```python
from build123d import *

# Parameters (mm, degrees)
SKETCH1_R           = 2.25
BOSS_EXTRUDE1_DEPTH = 30
SKETCH2_R           = 3.5
BOSS_EXTRUDE2_DEPTH = 2
BOSS_EXTRUDE2_TAPER = 6
CUT_EXTRUDE1_DEPTH  = 1


with BuildPart() as part:
    # Sketch1 → Boss-Extrude1 (new body)
    with BuildSketch(Plane.XY):
        Circle(SKETCH1_R)
    extrude(amount=BOSS_EXTRUDE1_DEPTH)

    # Sketch2 → Boss-Extrude2 (add)
    with BuildSketch(Plane(origin=(0, 0, 0), x_dir=(-1, 0, 0), z_dir=(0, 0, -1))):
        Circle(SKETCH2_R)
    extrude(amount=BOSS_EXTRUDE2_DEPTH, taper=BOSS_EXTRUDE2_TAPER)

    # Sketch3 → Cut-Extrude1 (cut)
    with BuildSketch(Plane(origin=(0, 0, -2), x_dir=(-1, 0, 0), z_dir=(0, 0, -1))):
        with BuildLine():
            Line((-0.4, 0.4), (-0.4, 3.065383332))
            ThreePointArc((-0.4, 3.065383332), (-0.341421356, 3.206804689), (-0.2, 3.265383332))
            Line((-0.2, 3.265383332), (0.2, 3.265383332))
            ThreePointArc((0.2, 3.265383332), (0.341421356, 3.206804689), (0.4, 3.065383332))
            Line((0.4, 3.065383332), (0.4, 0.4))
            Line((0.4, 0.4), (1.721973592, 0.4))
            ThreePointArc((1.721973592, 0.4), (1.863394949, 0.341421356), (1.921973592, 0.2))
            Line((1.921973592, 0.2), (1.921973592, -0.2))
            ThreePointArc((1.921973592, -0.2), (1.863394949, -0.341421356), (1.721973592, -0.4))
            Line((1.721973592, -0.4), (0.4, -0.4))
            Line((0.4, -0.4), (0.4, -3.065383332))
            ThreePointArc((0.4, -3.065383332), (0.341421356, -3.206804689), (0.2, -3.265383332))
            Line((0.2, -3.265383332), (-0.2, -3.265383332))
            ThreePointArc((-0.2, -3.265383332), (-0.341421356, -3.206804689), (-0.4, -3.065383332))
            Line((-0.4, -3.065383332), (-0.4, -0.4))
            Line((-0.4, -0.4), (-1.721973592, -0.4))
            ThreePointArc((-1.721973592, -0.4), (-1.863394949, -0.341421356), (-1.921973592, -0.2))
            Line((-1.921973592, -0.2), (-1.921973592, 0.2))
            ThreePointArc((-1.921973592, 0.2), (-1.863394949, 0.341421356), (-1.721973592, 0.4))
            Line((-1.721973592, 0.4), (-0.4, 0.4))
        make_face()
    extrude(amount=-CUT_EXTRUDE1_DEPTH, mode=Mode.SUBTRACT)


solid = part.part
```
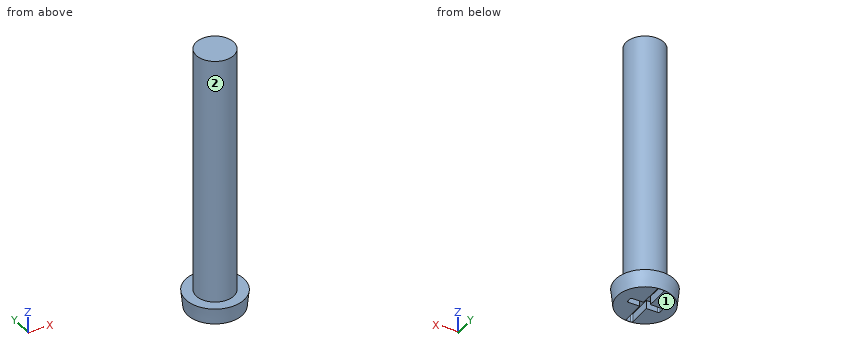
For this review, take the finished solid that the model builds, in its own axes (mm). Face numbers are marked on the shaded views. A direction names the side the tool comes from. Give positions to 0.01 mm unless a question says otherwise; leave off trailing zeros. Order: outer loops, then holes, each group sorted by start corner. A loop starts at its lowest first (then second) coordinate and runs counter-clockwise, first axis right, second up.
1) Take a section at A-A (z = 1.5). Give the boundary of the cut face in (x, y), then the cut area to 3 significant figures.
2) For the marked faces 1 and 2, list the 3-axis set-ups (+Z, -Z, +X, -X, +Y, -Y) from which the entire face can be reached by the end or side of a thin tool; tool diameter is ignored.
3) Insertion check: pin 1 (0.5 mm diameter, centred on x = 1, z = -1.5, fed in from +Y); pin 2 (0.8 mm diameter, centred on y = -2.5, z = -1.5, fed in from +X); pin 3 (0.8 mm diameter, centred on x = -1, z = -1.5, fed in from -Y). Each pin has a flat end and moves straight along its axis. Give the tip position at first contact, or say it passes through.
4) Wall thickness on line 1 (Z direction, x = 0.75, y = 2.5); line 2 (Z direction, x = 1.25, y = -0.25); line 3 (Y direction, x = 1, z = 14): over which ranges is each line inside the solid? List them lowest first.
Derived:
1. outline: circle Ø4.5 at (0, 0)
1. area: 15.9 mm2
2. face 1: -Z, +X, -X, +Y, -Y
2. face 2: +Z
3. pin 1: stops at y = 3.26
3. pin 2: stops at x = 2.6
3. pin 3: stops at y = -3.3
4. line 1: z = -2 to 0
4. line 2: z = -1 to 30
4. line 3: y = -2.02 to 2.02
